```python
from build123d import *

# Parameters (mm, degrees)
AUFSATZ_LINEAR_AUSTRAGEN1_DEPTH                      = 4
STIRNSENKUNG_F_R_M3_ZYLINDERSCHRAUBE_MIT_D           = 3.2
STIRNSENKUNG_F_R_M3_ZYLINDERSCHRAUBE_MIT_CBORE_D     = 5.8
STIRNSENKUNG_F_R_M3_ZYLINDERSCHRAUBE_MIT_CBORE_DEPTH = 2
M3_GEWINDEBOHRUNG1_D                                 = 2.5
M3_GEWINDEBOHRUNG1_DEPTH                             = 8.5
M3_GEWINDEBOHRUNG1_TIP                               = 0.751075774
M2_GEWINDEBOHRUNG1_D                                 = 1.6
M2_GEWINDEBOHRUNG1_DEPTH                             = 6
M2_GEWINDEBOHRUNG1_TIP                               = 0.480688495
SKIZZE3_W                                            = 65.5
SKIZZE3_H                                            = 33
SCHNITT_LINEAR_AUSTRAGEN1_DEPTH                      = 6
SCHNITT_LINEAR_AUSTRAGEN2_DEPTH                      = 9
VERRUNDUNG1_R                                        = 4


with BuildPart() as part:
    # Skizze2 → Aufsatz-Linear austragen1 (new body, symmetric)
    with BuildSketch(Plane(origin=(0, 0, 0), x_dir=(1, 0, 0), z_dir=(0, 0, -1))):
        Polygon((-100, 19.5), (-100, 5.5), (-88.5, 5.5), (-88.5, 0), (0, 0), (0, 19.5), align=None)
    extrude(amount=AUFSATZ_LINEAR_AUSTRAGEN1_DEPTH, both=True)

    # Stirnsenkung für  M3 Zylinderschraube mit Schlitz/Kreuzschlitz1 (through all)
    with Locations(Plane(origin=(0, -19.5, 0), x_dir=(-1, 0, 0), z_dir=(0, -1, 0))):
        with Locations((92.5, 0)):
            CounterBoreHole(STIRNSENKUNG_F_R_M3_ZYLINDERSCHRAUBE_MIT_D / 2, STIRNSENKUNG_F_R_M3_ZYLINDERSCHRAUBE_MIT_CBORE_D / 2, STIRNSENKUNG_F_R_M3_ZYLINDERSCHRAUBE_MIT_CBORE_DEPTH)

    # Spiegeln2: part across plane


with BuildPart() as part_1:
    add(part.part)
    add(part.part.mirror(Plane.ZX))

    # M3 Gewindebohrung1
    with Locations(Plane.ZY.offset(88.5)):
        with Locations((0, 0)):
            Hole(M3_GEWINDEBOHRUNG1_D / 2, depth=M3_GEWINDEBOHRUNG1_DEPTH)
            with Locations((0, 0, -(M3_GEWINDEBOHRUNG1_DEPTH + M3_GEWINDEBOHRUNG1_TIP / 2))):  # 118° drill point
                Cone(0, M3_GEWINDEBOHRUNG1_D / 2, M3_GEWINDEBOHRUNG1_TIP, mode=Mode.SUBTRACT)

    # M2 Gewindebohrung1
    with Locations(Plane.ZY.offset(100)):
        with Locations((0, 10), (0, -10)):
            Hole(M2_GEWINDEBOHRUNG1_D / 2, depth=M2_GEWINDEBOHRUNG1_DEPTH)
            with Locations((0, 0, -(M2_GEWINDEBOHRUNG1_DEPTH + M2_GEWINDEBOHRUNG1_TIP / 2))):  # 118° drill point
                Cone(0, M2_GEWINDEBOHRUNG1_D / 2, M2_GEWINDEBOHRUNG1_TIP, mode=Mode.SUBTRACT)

    # Spiegeln3: part across plane


with BuildPart() as part_2:
    add(part_1.part)
    add(part_1.part.mirror(Plane(origin=(0, 0, 0), x_dir=(0, 0, 1), z_dir=(1, 0, 0))))

    # Skizze3 → Schnitt-Linear austragen1 (cut)
    with BuildSketch(Plane.XY.offset(4)):
        with Locations((-34.25, 0)):
            Rectangle(SKIZZE3_W, SKIZZE3_H)
        with Locations((34.25, 0)):
            Rectangle(SKIZZE3_W, SKIZZE3_H)
    extrude(amount=-SCHNITT_LINEAR_AUSTRAGEN1_DEPTH, mode=Mode.SUBTRACT)

    # Skizze3<3> → Schnitt-Linear austragen2 (cut, through all)
    with BuildSketch(Plane.XY.offset(4)):
        with BuildLine():
            Line((-82.5, -4), (-74.5, -4))
            ThreePointArc((-74.5, -4), (-70.5, 0), (-74.5, 4))
            Line((-74.5, 4), (-82.5, 4))
            ThreePointArc((-82.5, 4), (-86.5, 0), (-82.5, -4))
        make_face()
        with BuildLine():
            Line((74.5, -4), (82.5, -4))
            ThreePointArc((82.5, -4), (86.5, 0), (82.5, 4))
            Line((82.5, 4), (74.5, 4))
            ThreePointArc((74.5, 4), (70.5, 0), (74.5, -4))
        make_face()
    extrude(amount=-SCHNITT_LINEAR_AUSTRAGEN2_DEPTH, mode=Mode.SUBTRACT)

    # Verrundung1
    verrundung1_edges = [part_2.edges().sort_by_distance(p)[0] for p in [
        (-67, 16.5, 1),
        (-67, -16.5, 1),
        (-1.5, -16.5, 1),
        (-1.5, 16.5, 1),
        (1.5, 16.5, 1),
        (1.5, -16.5, 1),
        (67, -16.5, 1),
        (67, 16.5, 1),
    ]]
    fillet(verrundung1_edges, radius=VERRUNDUNG1_R)


solid = part_2.part
```
Design review of the part built by this model. Coordinates are the model's own, in mm. A direction names the side the tool comes from. Coordinates: 2 decimals unless noted, no trailing zeros. Loops run counter-clockwise (first coordinate to the right, second up) from the corner with the lowest first, then second, coordinate; pieces in that order, holes last.
Q1. We need section A-A on x = -47. State the section outline as (y, z) points.
Reported:
outline: (-19.5, -4) - (19.5, -4) - (19.5, 4) - (16.5, 4) - (16.5, -2) - (-16.5, -2) - (-16.5, 4) - (-19.5, 4) - close
Q2. For pin 1 (3.5 mm diameter, centred on x = 92.5, z = 0, fed in from -Y); pin 2 (1.8 mm diameter, centred on y = -1, z = 2.5, fed in from +X); pin 3 (4 mm diameter, centred on x = 92.5, z = 0, fed in from +Y); pin 4 (1.8 mm diameter, centred on y = -10, z = 0, fed in from -X), all flat-tipped, find the tip position at first contact; note any pin that passes through.
Reported:
pin 1: stops at y = -17.5
pin 2: stops at x = 88.5
pin 3: stops at y = 17.5
pin 4: stops at x = -100
Q3. Tool access review of faces 1 (the face through (-94.3, 5.5, -0.1)), 2 (the face through (2.641, -15.297, 0.958)), 3 (the face through (-79, -4, 0)), 4 (the face through (94.3, 5.5, -0.1)): name each direction out of +Z, -Z, +X, -X, +Y, -Y from which nothing blocks a thin tool from reaching the whole face with its end or side.
Reported:
face 1: +Z, -Z, -X
face 2: +Z
face 3: +Z, -Z
face 4: +Z, -Z, +X
Q4. The part is to be moulded in two halves that separate along Z. For faces 5 (the face through (1, 0, 4)), 6 (the face through (-100, 13, 0)), 7 (the face through (-94, -17.5, 1)), say which applies: +Z half, -Z half, draft (parallel to the pull), parting line (faces both ways), or undercut.
Reported:
face 5: +Z half
face 6: draft
face 7: undercut
Q5. To check wall thickness, follow line 1 (Y direction, x = 95.5, z = 0); line 2 (X direction, y = -4.5, z = 1.5); line 3 (Y direction, x = 76, z = -1.75). State the ranges of each line that lie inside material, in increasing order.
Reported:
line 1: y = -19.5 to -10.8, -9.2 to -5.5, 5.5 to 9.2, 10.8 to 19.5
line 2: x = -88.5 to -67, -1.5 to 1.5, 67 to 88.5
line 3: y = -19.5 to -4, 4 to 19.5
